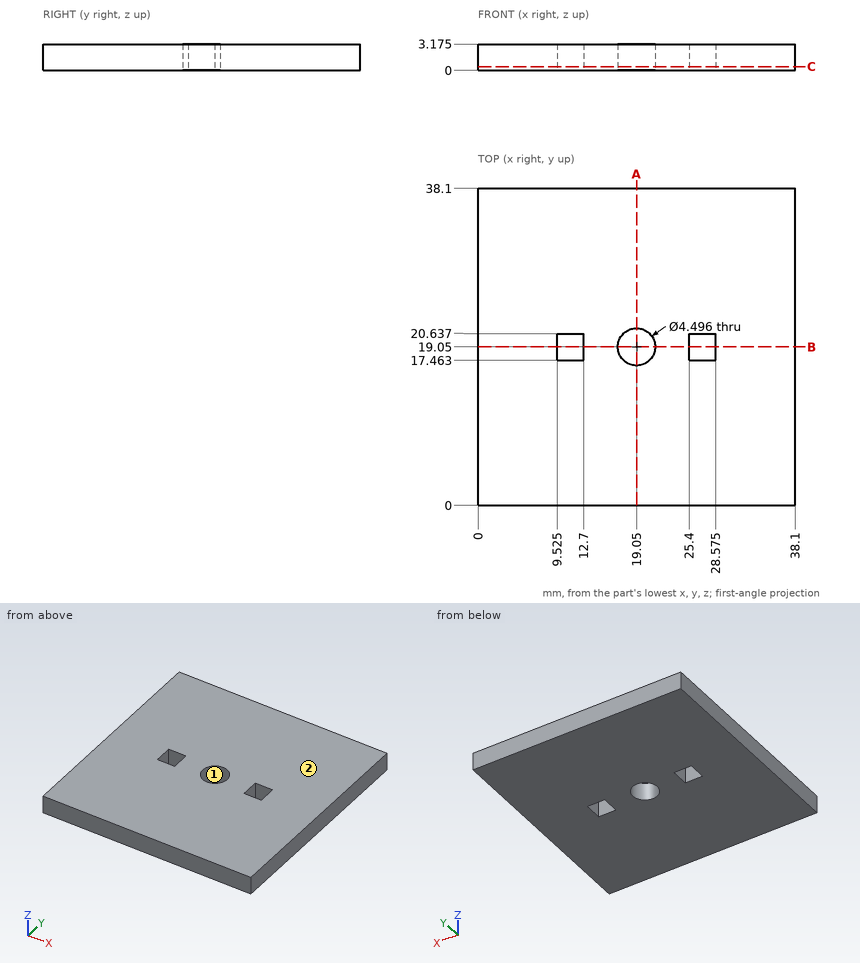
Input: dimensioned drawing with shaded views. Units: mm. Origin: part minimum x, y, z. Give positions to 0.01 mm unless a question says otherwise; leave off trailing zeros. Write each loop counter-clockwise with the first axis right and the second up, starting at its lowest first coordinate (ties: lowest second). Pieces come first, ordered by that corner, then holes.
Q1. Material intervals for probe 1 along Y at (x, z) = (19.05, 1.7); probe 2 along Y at (x, z) = (10, 0.5), sorted ascending.
Q2. Section B-B, the plane y = 19.05. Output: boundary loops of the cut face in (x, z) (1 decimal).
Q3. Section C-C, the plane z = 0.45. State how many separate pieces and enclosed holes the cut face has, plus the area to 3 significant figures.
Q4. Section A-A, the plane x = 19.05. Output: boundary loops of the cut face in (y, z) (1 decimal), plus the area to 3 significant figures.
Q5. Pull-direction query (X, two-part tool) for the marked faces 1 and 2; classes: pulls with the +X half, pulls with the -X half, needs draft (parallel to the pull), parting line crosses it, or undercut.
Filled in:
1. probe 1: y = 0 to 16.8, 21.3 to 38.1
1. probe 2: y = 0 to 17.46, 20.64 to 38.1
2. outline: (0, 0) - (9.5, 0) - (9.5, 3.2) - (0, 3.2) - close; (12.7, 0) - (16.8, 0) - (16.8, 3.2) - (12.7, 3.2) - close; (21.3, 0) - (25.4, 0) - (25.4, 3.2) - (21.3, 3.2) - close; (28.6, 0) - (38.1, 0) - (38.1, 3.2) - (28.6, 3.2) - close
3. separate pieces: 1
3. enclosed holes: 3
3. area: 1,420 mm2
4. outline: (0, 0) - (16.8, 0) - (16.8, 3.2) - (0, 3.2) - close; (21.3, 0) - (38.1, 0) - (38.1, 3.2) - (21.3, 3.2) - close
4. area: 107 mm2
5. face 1: undercut
5. face 2: needs draft
